The listing builds one solid part. Answer for the finished solid, in the listing's coordinates (mm). A direction names the side the tool comes from. Round coordinates to 2 decimals unless told otherwise and drop trailing zeros. Order: outer loops, then holes, each group sorted by start corner. A loop starts at its lowest first (then second) coordinate and runs counter-clockwise, first axis right, second up. Notation, with made-up numbers: (77.5, -13.5) - (111.5, -13.5) arc R13 ccw to (111.5, 4.5) - close; hole circle Ø1 at (11.25, 0.5). An arc over 180 degrees is marked (long way). Use CSV: the item, a comma, the result in double quotes. Start each with the question number.
Item 1: Determine the mould class of faces 1 (the flat face through (36, -19, -5)), 2 (the flat face through (41.83, -18.6, -2.46)), 3 (the flat face through (-39, -21.25, -2)) for opening direction Y: +Y half, -Y half, draft (parallel to the pull), parting line (faces both ways), or undercut.
Item 2: For faces 4 (the flat face through (39, -12.75, -2)), 5 (the flat face through (-40, -4, 0)), 6 (the flat face through (-42, -3, -5)), determine the directions among +Z, -Z, +X, -X, +Y, -Y from which every point of the face is accessible in a straight line to the end or side of a thin tool.
Item 3: Flat-ended cylindrical pins translate along their axes: P1, Ø8, axis at x = 53, y = -9, coming from the -Z side; P2, Ø2, axis at x = -38, y = -16, coming from the -Z side; P3, Ø3, axis at x = 39, y = -19, coming from the +Z side; P4, Ø5.5, axis at x = 39.5, z = -3, coming from the +Y side. Find the tip coordinate at first contact, or state that the pin passes through.
Item 4: Straight lines are drawn through the part: line 1 along X through (y, z) = (-1.3, 2.25); line 2 along Y through (x, z) = (39, 0.7); line 3 along Y through (x, z) = (-53, 2.7). For each, find the intervals that lie inside material, in ascending order. Write a range as [from, to].
Item 5: Find section D-D, the plane x = -25. Give the vertices of the cut face in (y, z).
Item 6: Find section A-A, the plane z = -2. Count the separate pieces of the cut face and the enclosed holes in it, plus the area to 3 significant figures.
Item 7: Find section B-B, the plane y = 14. Give the vertices of the cut face in (x, z).
```python
from build123d import *

# Parameters (mm, degrees)
SKETCH_1_W          = 120
SKETCH_1_H          = 50
SKETCH_1_R          = 2.5
EXTRUDE_2_DEPTH     = 5
SKETCH_4_R          = 2.5
CUT_EXTRUDE_1_DEPTH = 66.192024052
SKETCH_7_R          = 5
CUT_EXTRUDE_4_DEPTH = 2
EXTRUDE_3_DEPTH     = 5
SKETCH_11_W         = 5
SKETCH_11_H         = 12
CUT_EXTRUDE_5_DEPTH = 13
FILLET_3_R          = 6
SKETCH_12_W         = 5
SKETCH_12_H         = 12
CUT_EXTRUDE_6_DEPTH = 13
FILLET_4_R          = 6
CUT_EXTRUDE_7_DEPTH = 2


with BuildPart() as part:
    # 草图1 → 凸台-拉伸2 (new body)
    with BuildSketch(Plane.XY):
        Rectangle(SKETCH_1_W, SKETCH_1_H)
        with Locations((-53, -9)):
            Circle(SKETCH_1_R, mode=Mode.SUBTRACT)
        with Locations((53, -9)):
            Circle(SKETCH_1_R, mode=Mode.SUBTRACT)
    extrude(amount=EXTRUDE_2_DEPTH)

    # 草图4 → 切除-拉伸1 (cut, through all)
    with BuildSketch(Plane.XY):
        with Locations((-39, -1.3)):
            Circle(SKETCH_4_R)
        with Locations((-39, -17)):
            Circle(SKETCH_4_R)
        with Locations((39, -1.3)):
            Circle(SKETCH_4_R)
        with Locations((39, -17)):
            Circle(SKETCH_4_R)
    extrude(amount=CUT_EXTRUDE_1_DEPTH, mode=Mode.SUBTRACT)

    # 草图7 → 切除-拉伸4 (cut)
    with BuildSketch(Plane.XY.offset(5)):
        with Locations((-39, -1.3)):
            Circle(SKETCH_7_R)
        with Locations((-39, -17)):
            Circle(SKETCH_7_R)
        with Locations((39, -1.3)):
            Circle(SKETCH_7_R)
        with Locations((39, -17)):
            Circle(SKETCH_7_R)
    extrude(amount=-CUT_EXTRUDE_4_DEPTH, mode=Mode.SUBTRACT)

    # 草图9 → 凸台-拉伸3 (add)
    # profile 1 of 4: a face of its own
    with BuildSketch(Plane(origin=(0, 0, 0), x_dir=(-1, 0, 0), z_dir=(0, 0, -1))):
        Polygon((-34.092522712, -1.3), (-36.546261356, 2.95), (-41.453738644, 2.95), (-43.907477288, -1.3), (-41.453738644, -5.55), (-36.546261356, -5.55), align=None)
        Polygon((-35.24722325, -1.3), (-37.123611625, 1.95), (-40.876388375, 1.95), (-42.75277675, -1.3), (-40.876388375, -4.55), (-37.123611625, -4.55), align=None, mode=Mode.SUBTRACT)
    # profile 2 of 4: a face of its own
    with BuildSketch(Plane(origin=(0, 0, 0), x_dir=(-1, 0, 0), z_dir=(0, 0, -1))):
        Polygon((-34.092522712, -17), (-36.546261356, -12.75), (-41.453738644, -12.75), (-43.907477288, -17), (-41.453738644, -21.25), (-36.546261356, -21.25), align=None)
        Polygon((-35.24722325, -17), (-37.123611625, -13.75), (-40.876388375, -13.75), (-42.75277675, -17), (-40.876388375, -20.25), (-37.123611625, -20.25), align=None, mode=Mode.SUBTRACT)
    # profile 3 of 4: a face of its own
    with BuildSketch(Plane(origin=(0, 0, 0), x_dir=(-1, 0, 0), z_dir=(0, 0, -1))):
        Polygon((43.907477288, -1.3), (41.453738644, 2.95), (36.546261356, 2.95), (34.092522712, -1.3), (36.546261356, -5.55), (41.453738644, -5.55), align=None)
        Polygon((42.75277675, -1.3), (40.876388375, 1.95), (37.123611625, 1.95), (35.24722325, -1.3), (37.123611625, -4.55), (40.876388375, -4.55), align=None, mode=Mode.SUBTRACT)
    # profile 4 of 4: a face of its own
    with BuildSketch(Plane(origin=(0, 0, 0), x_dir=(-1, 0, 0), z_dir=(0, 0, -1))):
        Polygon((43.907477288, -17), (41.453738644, -12.75), (36.546261356, -12.75), (34.092522712, -17), (36.546261356, -21.25), (41.453738644, -21.25), align=None)
        Polygon((42.75277675, -17), (40.876388375, -13.75), (37.123611625, -13.75), (35.24722325, -17), (37.123611625, -20.25), (40.876388375, -20.25), align=None, mode=Mode.SUBTRACT)
    extrude(amount=EXTRUDE_3_DEPTH)

    # 草图11 → 切除-拉伸5 (cut)
    with BuildSketch(Plane(origin=(60, 0, 0), x_dir=(0, 0, -1), z_dir=(1, 0, 0))):
        with Locations((-2.5, -19)):
            Rectangle(SKETCH_11_W, SKETCH_11_H)
    extrude(amount=-CUT_EXTRUDE_5_DEPTH, mode=Mode.SUBTRACT)

    # 圆角3
    fillet_3_edges = [part.edges().sort_by_distance(p)[0] for p in [
        (47, -13, 2.5),
    ]]
    fillet(fillet_3_edges, radius=FILLET_3_R)

    # 草图12 → 切除-拉伸6 (cut)
    with BuildSketch(Plane.ZY.offset(60)):
        with Locations((2.5, -19)):
            Rectangle(SKETCH_12_W, SKETCH_12_H)
    extrude(amount=-CUT_EXTRUDE_6_DEPTH, mode=Mode.SUBTRACT)

    # 圆角4
    fillet_4_edges = [part.edges().sort_by_distance(p)[0] for p in [
        (-47, -13, 2.5),
    ]]
    fillet(fillet_4_edges, radius=FILLET_4_R)

    # 草图13 → 切除-拉伸7 (cut)
    with BuildSketch(Plane(origin=(0, 0, 0), x_dir=(-1, 0, 0), z_dir=(0, 0, -1))):
        Polygon((-49.24722325, -9), (-51.123611625, -5.75), (-54.876388375, -5.75), (-56.75277675, -9), (-54.876388375, -12.25), (-51.123611625, -12.25), align=None)
        Polygon((56.75277675, -9), (54.876388375, -5.75), (51.123611625, -5.75), (49.24722325, -9), (51.123611625, -12.25), (54.876388375, -12.25), align=None)
    extrude(amount=-CUT_EXTRUDE_7_DEPTH, mode=Mode.SUBTRACT)


solid = part.part
```
Worked out:
1,face 1,"draft"
1,face 2,"undercut"
1,face 3,"-Y half"
2,face 4,"-Z, +X, -X"
2,face 5,"-Z"
2,face 6,"-Z, +X, -X, +Y, -Y"
3,P1,"stops at z = 0"
3,P2,"passes through"
3,P3,"stops at z = 3"
3,P4,"stops at y = 2.95"
4,line 1,"x = [-60, -41.5], [-36.5, 36.5], [41.5, 60]"
4,line 2,"y = [-25, -19.5], [-14.5, -3.8], [1.2, 25]"
4,line 3,"y = [-13, -11.5], [-6.5, 25]"
5,outline,"(-25, 0) - (25, 0) - (25, 5) - (-25, 5) - close"
6,separate pieces,"4"
6,enclosed holes,"4"
6,area,"104 mm²"
7,outline,"(-60, 0) - (60, 0) - (60, 5) - (-60, 5) - close"
